```python
from build123d import *

# Parameters (mm, degrees)
F1_DEPTH = 25
F3_DEPTH = 60.001
F4_R     = 5
F5_W     = 13
F5_H     = 6
F6_DEPTH = 15
F7_R     = 4
F8_DEPTH = 25.001


with BuildPart() as f1:
    # F0 (on Front) → F1 (new body)
    with BuildSketch(Plane.XZ):
        Polygon((29.442134, 17.5), (-30.557866, 17.5), (-30.557866, -7.5), (-20.1, -7.5), (-20.1, 7.5), (-10, 7.5), (-10, -7.5), (10, -7.5), (10, 7.5), (20.1, 7.5), (11.439746, -7.5), (29.442134, -7.5), align=None)
        Polygon((-20.1, 7.5), (-20.1, -7.5), (-11.439746, -7.5), align=None)
    extrude(amount=F1_DEPTH)

    # F2 (on face) → F3 (cut, through all)
    with BuildSketch(Plane(origin=(-30.557866, 0, 0), x_dir=(0, -1, 0), z_dir=(-1, 0, 0))):
        Polygon((15, 12.5), (25, 12.5), (25, 17.5), (5, 17.5), align=None)
    extrude(amount=-F3_DEPTH, mode=Mode.SUBTRACT)

    # F4
    f4_edges = [f1.edges().sort_by_distance(p)[0] for p in [
        (-0.557866, -15, 12.5),
    ]]
    fillet(f4_edges, radius=F4_R)

    # F5 (on face) → F6 (cut)
    with BuildSketch(Plane(origin=(0, 0, -7.5), x_dir=(1, 0, 0), z_dir=(0, 0, -1))):
        with Locations((0, 12.5)):
            Rectangle(F5_W, F5_H)
    extrude(amount=-F6_DEPTH, mode=Mode.SUBTRACT)

    # F7 (on face) → F8 (cut, through all)
    with BuildSketch(Plane.XZ.offset(25)):
        Circle(F7_R)
    extrude(amount=-F8_DEPTH, mode=Mode.SUBTRACT)


solid = f1.part
```
Check sheet for the modelled part. Datum: model origin and axes. Units: mm. A direction names the side the tool comes from. Round coordinates to 2 decimals unless told otherwise and drop trailing zeros. Write each loop counter-clockwise with the first axis right and the second up, starting at its lowest first coordinate (ties: lowest second). Pieces come first, ordered by that corner, then holes. Notation, with made-up numbers: (-32, 63) -> (-11, 63) arc R22 cw to (-11, 87) -> close; hole circle Ø3 at (-3.5, 59.5). An arc over 180 degrees is marked (long way). One line per question, with ' | ' between items. Start each with the question number.
1. Sectioned sample at C-C, the plane y = -20.5. Record the cut outline in (x, z), then the cut area to 3 significant figures.
2. Release check for a two-part mould opening along X. For faces 6 (the face through (15, -12, 7.5)), 7 (the face through (29.442, -12, 2)), 8 (the face through (-1, -21, 12.5)) record: +X half, -X half, draft (parallel to the pull), parting line (faces both ways), or undercut.
3. Sectioned sample at D-D, the plane x = 7.5. Record the cut outline in (y, z).
4. Set-up check for faces 1 (the face through (6.5, -12, 0)), 2 (the face through (15.83, -12.325, 0.105)), 3 (the face through (-1, -9.4, 15.3)), 4 (the face through (-30.558, -12, 2)), 5 (the face through (-10, -12, 0)): record each of +Z, -Z, +X, -X, +Y, -Y from which the full face is reachable in a straight line by a thin tool's end or side.
5. Scan lines: line 1 along Z through (x, y) = (0, -2.75); line 2 along X through (y, z) = (-20, 5.75); line 3 along X through (y, z) = (-7.75, -2). Record each from-to range of solid material in increasing order. Write a range as from..to.
6. Sectioned sample at A-A, the plane x = 0. Record the cut outline in (y, z), then the cut area to 3 significant figures.
7. Depth check by flat-ended pin: pin 1 (6 mm diameter, centred on x = 3, y = -6.5, fed in from +Z); pin 2 (2 mm diameter, centred on x = 5, y = -17, fed in from +Z). Enter the tip coordinate at first touch or a pass-through.
8. Sectioned sample at B-B, the plane z = 6. Record the cut outline in (x, y), then the cut area to 3 significant figures.
Taken from the geometry:
1) outline: (-30.56, -7.5) -> (-11.44, -7.5) -> (-20.1, 7.5) -> (-10, 7.5) -> (-10, -7.5) -> (10, -7.5) -> (10, 7.5) -> (20.1, 7.5) -> (11.44, -7.5) -> (29.44, -7.5) -> (29.44, 12.5) -> (-30.56, 12.5) -> close; hole circle Ø8 at (0, 0) | area: 977 mm^2
2) face 6: undercut | face 7: +X half | face 8: draft
3) outline: (-25, -7.5) -> (0, -7.5) -> (0, 17.5) -> (-5, 17.5) -> (-13.94, 13.03) arc R5 cw to (-16.18, 12.5) -> (-25, 12.5) -> close
4) face 1: -Z | face 2: +Y, -Y | face 3: +Z, +X, -X, -Y | face 4: +Z, -Z, -X, +Y, -Y | face 5: -Z, +Y, -Y
5) line 1: z = -7.5..-4, 4..17.5 | line 2: x = -30.56..-19.09, -10..10, 19.09..29.44 | line 3: x = -30.56..-14.62, -10..-3.46, 3.46..10, 14.62..29.44
6) outline: (-25, -7.5) -> (-15.5, -7.5) -> (-15.5, -4) -> (-25, -4) -> close; (-25, 4) -> (-15.5, 4) -> (-15.5, 7.5) -> (-9.5, 7.5) -> (-9.5, 4) -> (0, 4) -> (0, 17.5) -> (-5, 17.5) -> (-13.94, 13.03) arc R5 cw to (-16.18, 12.5) -> (-25, 12.5) -> close; (-9.5, -7.5) -> (0, -7.5) -> (0, -4) -> (-9.5, -4) -> close | area: 308 mm^2
7) pin 1: stops at z = 17.5 | pin 2: stops at z = 12.5
8) outline: (-30.56, -25) -> (-19.23, -25) -> (-19.23, 0) -> (-30.56, 0) -> close; (-10, -25) -> (10, -25) -> (10, 0) -> (-10, 0) -> close; (19.23, -25) -> (29.44, -25) -> (29.44, 0) -> (19.23, 0) -> close; hole (-6.5, -15.5) -> (6.5, -15.5) -> (6.5, -9.5) -> (-6.5, -9.5) -> close | area: 960 mm^2
